```python
from build123d import *

# Parameters (mm, degrees)
CIRPATTERN1_COUNT = 3


with BuildPart() as part:
    # Sketch1 → Revolve1 (revolve)
    with BuildSketch(Plane(origin=(0, 0, 0), x_dir=(-1, 0, 0), z_dir=(0, 0, -1)), mode=Mode.PRIVATE) as revolve1_sk:
        Polygon((-65, 262.227948901), (-40, 262.227948901), (-40, -124.772051099), (-26.75, -124.772051099), (-26.75, -212.772051099), (0, -212.772051099), (0, 262.227948901), (0, 357.227948901), (-40, 357.227948901), (-40, 291.733137356), (-65, 274.227948901), align=None)
    revolve(revolve1_sk.sketch.rotate(Axis((0, 262.227948901, 0), (0, 1, 0)), 270), axis=Axis((0, 262.227948901, 0), (0, 1, 0)))

    # Sketch4 → M8x1.0 Tapped Hole1 (revolve, cut)
    with BuildSketch(Plane(origin=(0, -212.772051099, -16), x_dir=(0, 0, -1), z_dir=(1, 0, 0))):
        Polygon((0, 0), (0, 21.103012167), (3.5, 19), (3.5, 0), align=None)
    m8x1_0_tapped_hole1 = revolve(axis=Axis((0, -219.122051099, -16), (0, 1, 0)), mode=Mode.SUBTRACT)

    # CirPattern1: M8x1.0 Tapped Hole1 ×3 about axis
    cirpattern1_axis = Axis((0, 0, 0), (0, 1, 0))
    for i in range(1, CIRPATTERN1_COUNT):
        add(m8x1_0_tapped_hole1.rotate(cirpattern1_axis, i * 360 / CIRPATTERN1_COUNT), mode=Mode.SUBTRACT)


solid = part.part
```
Check sheet for the modelled part. Datum: model origin and axes. Units: mm. A direction names the side the tool comes from. Round coordinates to 2 decimals unless told otherwise and drop trailing zeros. Write each loop counter-clockwise with the first axis right and the second up, starting at its lowest first coordinate (ties: lowest second). Pieces come first, ordered by that corner, then holes. Notation, with made-up numbers: M 31.5,-14 L 71.5,-14 A10 ccw 71.5,-9 Z; hole C -15,27.5 d5. An arc over 180 degrees is marked long. Write item = value, one per line. Start each with the question number.
1. Scan lines: line 1 (X direction, y = -202.5, z = 8); line 2 (Y direction, x = 36.5, z = 0); line 3 (X direction, y = -70, z = -9.5). Record each from-to range of solid material in increasing order. Write a range as [from, to].
2. Section check A-A, the plane y = -169.5. Record the cut outline in (x, z), then the cut area to 3 significant figures.
3. Section check B-B, the plane y = -25.5. Record the cut outline in (x, z).
4. Gauge pin test, flat ends, axial feed: pin 1 (4 mm diameter, centred on x = 24.5, z = 42.5, fed in from -Y); pin 2 (4 mm diameter, centred on y = 286.5, z = -19.5, fed in from -X); pin 3 (12 mm diameter, centred on x = 33.5, y = 30, fed in from -Z); pin 4 (8 mm diameter, centred on x = 0, z = -16, fed in from -Y). Record the tip position at first contact, or that the pin passes through.
5. Tool access check on faces 1 (the cylindrical face through (-16.277, -169.388, -21.228)), 2 (the cylindrical face through (19.52, 268.14, 62)), 3 (the cylindrical face through (-39.05, 324.02, -8.67)). Record the directions out of +Z, -Z, +X, -X, +Y, -Y that give a thin tool (end or side, any length) a straight path to the whole face; none if there is none.
Results found:
q1.line_1 = [-25.53, -17.36], [-10.36, 10.36], [17.36, 25.53]
q1.line_2 = [-124.77, 357.23]
q1.line_3 = [-38.86, 38.86]
q2.outline = C 0,0 d53.5
q2.area = 2,250 mm^2
q3.outline = C 0,0 d80
q4.pin_1 = 262.23
q4.pin_2 = -46.51
q4.pin_3 = -29.05
q4.pin_4 = -212.77
q5.face_1 = -Y
q5.face_2 = +Y, -Y
q5.face_3 = +Y
